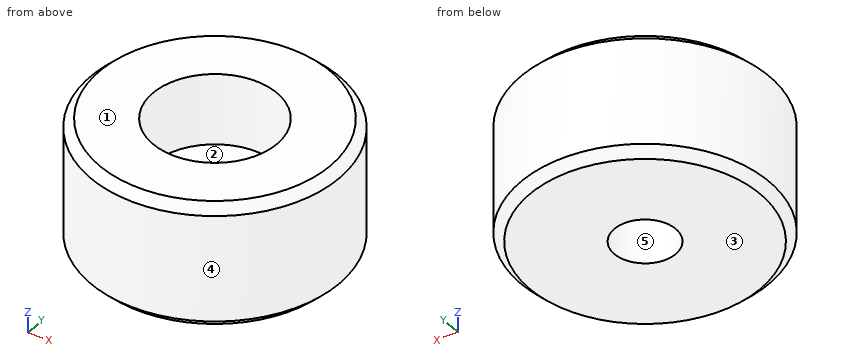
Autodesk Inventor part; units mm, degrees
ref_plane "YZ Plane" through (0, 0, 0) normal (1, 0, 0) x (0, 1, 0)
ref_plane "XZ Plane" through (0, 0, 0) normal (0, 1, 0) x (-1, 0, 0)
ref_plane "XY Plane" through (0, 0, 0) normal (0, 0, 1) x (1, 0, 0)
sketch "Sketch1" plane through (0, 0, 0) normal (0, 0, 1) x (1, 0, 0)
  circle A0 centre (0, 0) radius 3.5
  dimension "d0" = 7
extrude "Extrusion1" add sketch "Sketch1" along normal blind 3.5
hole "Hole1" at (0, 0, 0) direction (0, 0, 1) diameter 1.7294 depth 10 tip angle 118
chamfer "Chamfer1" distance 0.25 angle 45 2 edges at (-3.5, 0, 3.5) (-3.5, 0, 0)
sketch "Sketch2" plane through (0, 0, 3.5) normal (0, 0, 1) x (1, 0, 0)
  circle A0 centre (0, 0) radius 1.75
  dimension "d13" = 3.5
extrude "Extrusion2" cut sketch "Sketch2" against normal blind 2
properties part number "Cover of port"
Check sheet for the modelled part. Datum: model origin and axes. Units: mm. Face numbers are marked on the shaded views. A direction names the side the tool comes from. Give positions to 0.01 mm unless a question says otherwise; leave off trailing zeros. Order: outer loops, then holes, each group sorted by start corner. A loop starts at its lowest first (then second) coordinate and runs counter-clockwise, first axis right, second up. Notation, with made-up numbers: (5.5, 13) -> (22.5, 13) arc R32 cw to (22.5, 51) -> close; hole circle Ø10 at (6, -25.75). An arc over 180 degrees is marked (long way). Use CSV: the item, a comma, the result in double quotes. Start each with the question number.
1) Set-up check for the marked faces 1 and 2: record each of +Z, -Z, +X, -X, +Y, -Y from which the full face is reachable in a straight line by a thin tool's end or side.
2) Sectioned sample at C-C, the plane z = 0.7. Record the boundary of the cut face in (x, y).
3) Sectioned sample at B-B, the plane z = 1.7. Record the boundary of the cut face in (x, y).
4) Mould release check, pull along Y, two halves, no side actions. Record for the marked faces 3, 4 and 5: released by +Y, released by -Y, zero draft, split by the parting line, or undercut.
5) Go/stop test with flat-tipped pins: P1, Ø1, axis at x = 2, z = 3, coming from the -Y side; P2, Ø2, axis at y = 1.5, z = 0.5, coming from the -X side; P3, Ø2, axis at y = -1.5, z = 3, coming from the +X side. Record where each tip stops, or that it passes through.
6) Material ranges on line 1 (Y direction, x = 0, z = 1.05); line 2 (Y direction, x = 0, z = 2.9); line 3 (X direction, y = 0.5, z = 1.7), recorded low to high. Write a range as from..to.
7) Sectioned sample at A-A, the plane x = 0. Record the boundary of the cut face in (y, z), plus the area to 3 significant figures.
Recorded:
1,face 1,"+Z, +X, -X, +Y, -Y"
1,face 2,"+Z"
2,outline,"circle Ø7 at (0, 0); hole circle Ø1.73 at (0, 0)"
3,outline,"circle Ø7 at (0, 0); hole circle Ø3.5 at (0, 0)"
4,face 3,"zero draft"
4,face 4,"split by the parting line"
4,face 5,"undercut"
5,P1,"y = -3.16"
5,P2,"x = -3.46"
5,P3,"x = 3.46"
6,line 1,"-3.5..-0.86, 0.86..3.5"
6,line 2,"-3.5..-1.75, 1.75..3.5"
6,line 3,"-3.46..-1.68, 1.68..3.46"
7,outline,"(-3.5, 0.25) -> (-3.25, 0) -> (-0.86, 0) -> (-0.86, 1.5) -> (-1.75, 1.5) -> (-1.75, 3.5) -> (-3.25, 3.5) -> (-3.5, 3.25) -> close; (0.86, 0) -> (3.25, 0) -> (3.5, 0.25) -> (3.5, 3.25) -> (3.25, 3.5) -> (1.75, 3.5) -> (1.75, 1.5) -> (0.86, 1.5) -> close"
7,area,"14.8 mm2"
